Could you check a few things on this drawing? It's one solid part, dimensions in mm from its lowest x, y, z. A direction names the side the tool comes from. Round coordinates to 2 decimals unless told otherwise and drop trailing zeros. Write each loop counter-clockwise with the first axis right and the second up, starting at its lowest first coordinate (ties: lowest second). Pieces come first, ordered by that corner, then holes. Notation, with made-up numbers: (8.25, -30.75) - (37.25, -30.75) arc R23 cw to (37.25, -3.75) - close; hole circle Ø10 at (61.25, 82). An arc over 180 degrees is marked (long way). Write item = value, one per line. Start each with the question number.
Item 1: Thinking about a two-plate mould opening in Z: for the marked faces 1, 2 and 3, which applies, pulls with the +Z half, pulls with the -Z half, needs draft (parallel to the pull), parting line crosses it, or undercut?
Item 2: Which directions (+Z, -Z, +X, -X, +Y, -Y) give clear straight access to the entire face, cutting with the end or side of a thin tool? Please do the marked faces 4 and 5.
Item 3: If we section it at A-A (z = 38): Please give me the cut outline in (x, y).
Item 4: If I drill on line 1 along X through (y, z) = (47, 135.5); line 2 along Y through (x, z) = (98, 135); line 3 along Z through (x, y) = (44, 35), over which ranges is the centre line in solid material (lowest first)? Write a range as [from, to].
Item 5: For P1, Ø3, axis at x = 98, z = 35, coming from the -Y side; P2, Ø3, axis at x = 86.5, z = 15.5, coming from the +Y side, each with a flat end and sliding along its axis, tell me the tip position at first contact or that it passes through.
Item 6: If we section it at B-B (y = 20): Please give me the cut outline in (x, z).
Item 7: If we section it at D-D (z = 85): Please give me the cut outline in (x, y).
Item 8: If we section it at C-C (y = 52): Please give me the cut outline in (x, z), and give its area (3 significant figures).
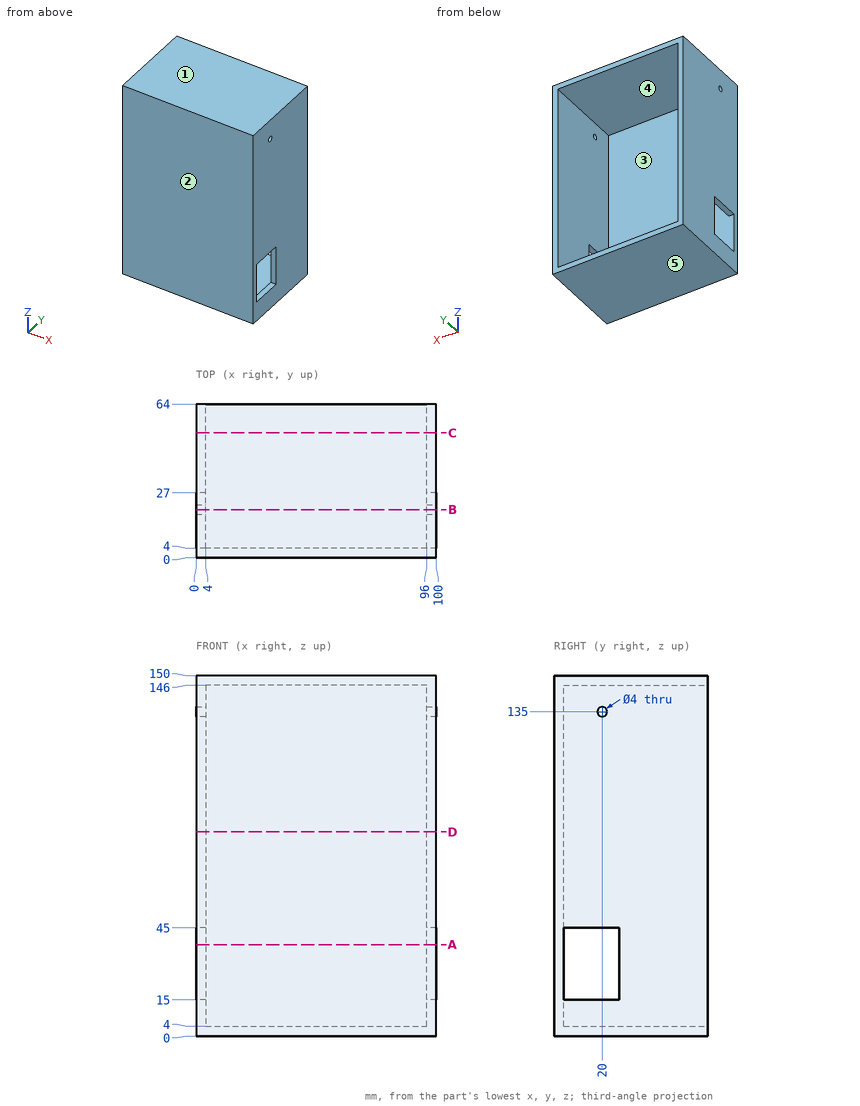
Reply:
q1.face_1 = pulls with the +Z half
q1.face_2 = needs draft
q1.face_3 = undercut
q2.face_4 = +Y
q2.face_5 = -Z, +X, -X, +Y, -Y
q3.outline = (0, 0) - (100, 0) - (100, 4) - (0, 4) - close; (0, 27) - (4, 27) - (4, 64) - (0, 64) - close; (96, 27) - (100, 27) - (100, 64) - (96, 64) - close
q4.line_1 = [0, 4], [96, 100]
q4.line_2 = [0, 18], [22, 64]
q4.line_3 = [0, 4], [146, 150]
q5.P1 = 0
q5.P2 = 4
q6.outline = (0, 0) - (100, 0) - (100, 15) - (96, 15) - (96, 4) - (4, 4) - (4, 15) - (0, 15) - close; (0, 45) - (4, 45) - (4, 133) - (0, 133) - close; (0, 137) - (4, 137) - (4, 146) - (96, 146) - (96, 137) - (100, 137) - (100, 150) - (0, 150) - close; (96, 45) - (100, 45) - (100, 133) - (96, 133) - close
q7.outline = (0, 0) - (100, 0) - (100, 64) - (96, 64) - (96, 4) - (4, 4) - (4, 64) - (0, 64) - close
q8.outline = (0, 0) - (100, 0) - (100, 150) - (0, 150) - close; hole (4, 4) - (96, 4) - (96, 146) - (4, 146) - close
q8.area = 1,940 mm2
